Work out the finished part from the listing and answer in its coordinate system (mm). A direction names the side the tool comes from. Round coordinates to 2 decimals unless told otherwise and drop trailing zeros. Write each loop counter-clockwise with the first axis right and the second up, starting at its lowest first coordinate (ties: lowest second). Pieces come first, ordered by that corner, then holes. Notation, with made-up numbers: (23.5, 61) -> (37.5, 61) arc R19 cw to (37.5, 78) -> close; hole circle Ø4 at (69.25, 53). An arc over 180 degrees is marked (long way). One line per item, written item: value.
```python
from build123d import *

# Parameters (mm, degrees)
BOSS_EXTRUDE1_DEPTH = 127
FILLET1_R           = 2.54
SKETCH2_R           = 4.7625
CUT_EXTRUDE1_DEPTH  = 6.35
SKETCH3_R           = 2.38125
CUT_EXTRUDE2_DEPTH  = 6.35


with BuildPart() as part:
    # Sketch1 → Boss-Extrude1 (new body)
    with BuildSketch(Plane(origin=(0, 0, 0), x_dir=(0, 0, -1), z_dir=(1, 0, 0))):
        Polygon((0, 0), (0, 101.6), (6.35, 101.6), (6.35, 6.35), (101.6, 6.35), (101.6, 0), align=None)
    extrude(amount=BOSS_EXTRUDE1_DEPTH)

    # Fillet1
    fillet1_edges = [part.edges().sort_by_distance(p)[0] for p in [
        (63.5, 6.35, -6.35),
    ]]
    fillet(fillet1_edges, radius=FILLET1_R)

    # Sketch2 → Cut-Extrude1 (cut)
    with BuildSketch(Plane(origin=(0, 0, -6.35), x_dir=(-1, 0, 0), z_dir=(0, 0, -1))):
        with Locations((-63.5, 70.696666667)):
            Circle(SKETCH2_R)
        with Locations((-63.5, 39.793333249)):
            Circle(SKETCH2_R)
    extrude(amount=-CUT_EXTRUDE1_DEPTH, mode=Mode.SUBTRACT)

    # Sketch3 → Cut-Extrude2 (cut)
    with BuildSketch(Plane(origin=(0, 6.35, 0), x_dir=(1, 0, 0), z_dir=(0, 1, 0))):
        with Locations((38.1, 80.645)):
            Circle(SKETCH3_R)
        with Locations((88.9, 80.645)):
            Circle(SKETCH3_R)
        with Locations((38.1, 29.845)):
            Circle(SKETCH3_R)
        with Locations((88.9, 29.845)):
            Circle(SKETCH3_R)
    extrude(amount=-CUT_EXTRUDE2_DEPTH, mode=Mode.SUBTRACT)


solid = part.part
```
(1) Find section D-D on z = -49. Give the vertices of the cut face in (x, y), plus the area to 3 significant figures.
Reported:
outline: (0, 0) -> (127, 0) -> (127, 6.35) -> (0, 6.35) -> close
area: 806 mm2
(2) Find section C-C on y = 73.5. Give the vertices of the cut face in (x, z).
Reported:
outline: (0, -6.35) -> (59.65, -6.35) -> (59.65, 0) -> (0, 0) -> close; (67.35, -6.35) -> (127, -6.35) -> (127, 0) -> (67.35, 0) -> close
(3) Find section B-B on x = 54. Give the vertices of the cut face in (y, z), plus the area to 3 significant figures.
Reported:
outline: (0, -101.6) -> (6.35, -101.6) -> (6.35, -8.89) arc R2.54 cw to (8.89, -6.35) -> (101.6, -6.35) -> (101.6, 0) -> (0, 0) -> close
area: 1,250 mm2
(4) Find section A-A on x = 38.1. Give the vertices of the cut face in (y, z).
Reported:
outline: (0, -101.6) -> (6.35, -101.6) -> (6.35, -83.03) -> (0, -83.03) -> close; (0, -78.26) -> (6.35, -78.26) -> (6.35, -32.23) -> (0, -32.23) -> close; (0, -27.46) -> (6.35, -27.46) -> (6.35, -8.89) arc R2.54 cw to (8.89, -6.35) -> (101.6, -6.35) -> (101.6, 0) -> (0, 0) -> close
(5) For a pull along Z with two mould halves and no side action, classify faces 1 (the face through (91.17, 3.22, -30.56)), 2 (the face through (91.17, 3.22, -81.36)), 3 (the face through (63, 56, -6.35)), 4 (the face through (127, 6, -28)) as pulls with the +Z half, pulls with the -Z half, needs draft (parallel to the pull), parting line crosses it, or undercut.
Reported:
face 1: undercut
face 2: undercut
face 3: pulls with the -Z half
face 4: needs draft
(6) Flat-ended cylindrical pins translate along their axes: pin 1 Ø8 at (x, y) = (67.5, 53.5) entering from -Z; pin 2 Ø4 at (x, z) = (38.1, -80.645) entering from +Y; pin 3 Ø1 at (x, z) = (97, -30) entering from +Y; pin 4 Ø1.5 at (x, z) = (62, -33.5) entering from -Y. Find the tip coordinate at first contact, or state that the pin passes through.
Reported:
pin 1: stops at z = -6.35
pin 2: passes through
pin 3: stops at y = 6.35
pin 4: stops at y = 0
(7) Consider probe 1 along Y at (x, z) = (63, -3); probe 2 along Z at (x, y) = (38.1, 3.5); probe 3 along Y at (x, z) = (63.5, -2). Determine where each line is inside the solid, lowest interval first.
Reported:
probe 1: y = 0 to 35.06, 44.53 to 65.96, 75.43 to 101.6
probe 2: z = -101.6 to -83.03, -78.26 to -32.23, -27.46 to 0
probe 3: y = 0 to 35.03, 44.56 to 65.93, 75.46 to 101.6
(8) A tool of negligible diameter and unlimited length cuts with its end or side. For faces 5 (the face through (40.37, 3.22, -30.56)), 6 (the face through (63, 6.35, -55)), from which of +Z, -Z, +X, -X, +Y, -Y can it reach the whole face along a straight path? Write none if from no direction.
Reported:
face 5: +Y, -Y
face 6: -Z, +X, -X, +Y
